Design review of the part built by this model. Coordinates are the model's own, in mm. A direction names the side the tool comes from. Coordinates: 2 decimals unless noted, no trailing zeros. Order: outer loops, then holes, each group sorted by start corner. A loop starts at its lowest first (then second) coordinate and runs counter-clockwise, first axis right, second up. Notation, with made-up numbers: M 6.5,24.25 L 31.5,24.25 A16 ccw 31.5,33.25 Z; hole C 46.5,67.25 d11. An arc over 180 degrees is marked long. Use CSV: the item, a comma, the result in double quotes.
```python
from build123d import *

# Parameters (mm, degrees)
SKETCH1_R                = 9.525
BOSS_EXTRUDE1_DEPTH      = 116.84
BOSS_EXTRUDE1_DEPTH_BACK = 51.562
SKETCH1_3_R              = 9.525
BOSS_EXTRUDE2_DEPTH      = 152.4


with BuildPart() as part:
    # Sketch1 → Boss-Extrude1 (new body, two sides)
    with BuildSketch(Plane.XY) as boss_extrude1_sk:
        Circle(SKETCH1_R)
        Polygon((-12.7, 7.332348419), (-12.7, -7.332348419), (0, -14.664696837), (12.7, -7.332348419), (12.7, 7.332348419), (0, 14.664696837), align=None)
        Circle(SKETCH1_R, mode=Mode.SUBTRACT)
    extrude(amount=BOSS_EXTRUDE1_DEPTH)
    extrude(boss_extrude1_sk.sketch, amount=-BOSS_EXTRUDE1_DEPTH_BACK)

    # Sketch1_3 → Boss-Extrude2 (add, symmetric)
    with BuildSketch(Plane.XY):
        Circle(SKETCH1_3_R)
    extrude(amount=BOSS_EXTRUDE2_DEPTH, both=True)


solid = part.part
```
(1) Add section C-C on x = -3.75. State the section outline as (y, z) points, and give its area (3 significant figures).
The answers:
outline,"M -12.5,-51.56 L -8.76,-51.56 L -8.76,-152.4 L 8.76,-152.4 L 8.76,-51.56 L 12.5,-51.56 L 12.5,116.84 L 8.76,116.84 L 8.76,152.4 L -8.76,152.4 L -8.76,116.84 L -12.5,116.84 Z"
area,"6,600 mm2"
(2) Add section B-B on z = 70. State the section outline as (x, y) points.
The answers:
outline,"M -12.7,-7.33 L 0,-14.66 L 12.7,-7.33 L 12.7,7.33 L 0,14.66 L -12.7,7.33 Z"
(3) Add section A-A on y = 0. State the section outline as (x, z) points (3 decimals).
The answers:
outline,"M -12.7,-51.562 L -9.525,-51.562 L -9.525,-152.4 L 9.525,-152.4 L 9.525,-51.562 L 12.7,-51.562 L 12.7,116.84 L 9.525,116.84 L 9.525,152.4 L -9.525,152.4 L -9.525,116.84 L -12.7,116.84 Z"
(4) Wall thickness on probe 1 along Z at (x, y) = (2.5, 9.5); probe 2 along X at (y, z) = (-13.25, -19.5); probe 3 along Y at (x, z) = (-4.75, 33.5): over which ranges is each line inside the solid? List them lowest first.
The answers:
probe 1,"z = -51.56 to 116.84"
probe 2,"x = -2.45 to 2.45"
probe 3,"y = -11.92 to 11.92"
(5) For faces 1 (the face through (0, 0, -152.4)), 2 (the face through (0, -10, 116.84)), 3 (the face through (-7.559, -5.796, -101.275)), list the 3-axis set-ups (+Z, -Z, +X, -X, +Y, -Y) from which the entire face can be reached by the end or side of a thin tool; tool diameter is ignored.
The answers:
face 1,"-Z, +X, -X, +Y, -Y"
face 2,"+Z"
face 3,"-Z"
(6) Clearance check with flat-ended pins moving along their axes: P1, Ø6, axis at y = -6, z = -79, coming from the +X side; P2, Ø4, axis at x = 9, y = -8.5, coming from the -Z side; P3, Ø1, axis at x = 2, z = 23, coming from the +Y side. State where each tip first meets the part, or that it passes through.
The answers:
P1,"stops at x = 9.04"
P2,"stops at z = -51.56"
P3,"stops at y = 13.8"
